CAD build for the part. Positions are in the model's coordinates, mm. Coordinates: 2 decimals unless noted, no trailing zeros. Loops run counter-clockwise (first coordinate to the right, second up) from the corner with the lowest first, then second, coordinate; pieces in that order, holes last. Notation, with made-up numbers: (-3, 73.25) - (21, 73.25) arc R34 ccw to (21, 104.25) - close; hole circle Ø1 at (36, 39). An arc over 180 degrees is marked (long way). Put each result on its own line as item: value.
```python
from build123d import *

# Parameters (mm, degrees)
SKETCH1_W           = 198
SKETCH1_H           = 230
SKETCH1_W_2         = 166
SKETCH1_H_2         = 210
BOSS_EXTRUDE1_DEPTH = 3
SKETCH2_W           = 7.09740754
SKETCH2_H           = 24
SKETCH2_W_2         = 5.8
SKETCH2_H_2         = 9.8
CUT_EXTRUDE1_DEPTH  = 3


with BuildPart() as part:
    # Sketch1 → Boss-Extrude1 (new body)
    with BuildSketch(Plane(origin=(0, 0, 0), x_dir=(1, 0, 0), z_dir=(0, 1, 0))):
        with Locations((99, 115)):
            Rectangle(SKETCH1_W, SKETCH1_H)
        with Locations((99, 115)):
            Rectangle(SKETCH1_W_2, SKETCH1_H_2, mode=Mode.SUBTRACT)
    extrude(amount=BOSS_EXTRUDE1_DEPTH)

    # Sketch2 → Cut-Extrude1 (cut)
    with BuildSketch(Plane(origin=(0, 3, 0), x_dir=(1, 0, 0), z_dir=(0, 1, 0))):
        with Locations((12.45129623, 120)):
            Rectangle(SKETCH2_W, SKETCH2_H)
        with Locations((191.99740754, 10.279523389)):
            Rectangle(SKETCH2_W_2, SKETCH2_H_2)
        with Locations((185.54870377, 110)):
            Rectangle(SKETCH2_W, SKETCH2_H)
        with Locations((191.99740754, 219.720476611)):
            Rectangle(SKETCH2_W_2, SKETCH2_H_2)
        with Locations((6.00259246, 219.720476611)):
            Rectangle(SKETCH2_W_2, SKETCH2_H_2)
        with Locations((6.00259246, 10.279523389)):
            Rectangle(SKETCH2_W_2, SKETCH2_H_2)
    extrude(amount=-CUT_EXTRUDE1_DEPTH, mode=Mode.SUBTRACT)


solid = part.part
```
Q1. Slice it at B-B, the plane z = -115.5. Give the cut face in (x, y), then the cut area to 3 significant figures.
Determined:
outline: (0, 0) - (8.9, 0) - (8.9, 3) - (0, 3) - close; (189.1, 0) - (198, 0) - (198, 3) - (189.1, 3) - close
area: 53.4 mm2
Q2. Wall check: L1, parallel to X at y = 0.3, z = -13.5; L2, parallel to Z at x = 17, y = 2.2; L3, parallel to X at y = 1.1, z = -39.5. Give the ranges that are in metal, low to high. Write a range as from..to.
Determined:
L1: 0..3.1, 8.9..16, 182..189.1, 194.9..198
L2: -230..-220, -10..0
L3: 0..16, 182..198
Q3. Slice it at C-C, the plane y = 1.9. State how many separate pieces and enclosed holes the cut face has, then the cut area to 3 significant figures.
Determined:
separate pieces: 1
enclosed holes: 5
area: 10,100 mm2
Q4. Slice it at A-A, the plane x = 168. Give the cut face in (y, z).
Determined:
outline: (0, -230) - (3, -230) - (3, -220) - (0, -220) - close; (0, -10) - (3, -10) - (3, 0) - (0, 0) - close
